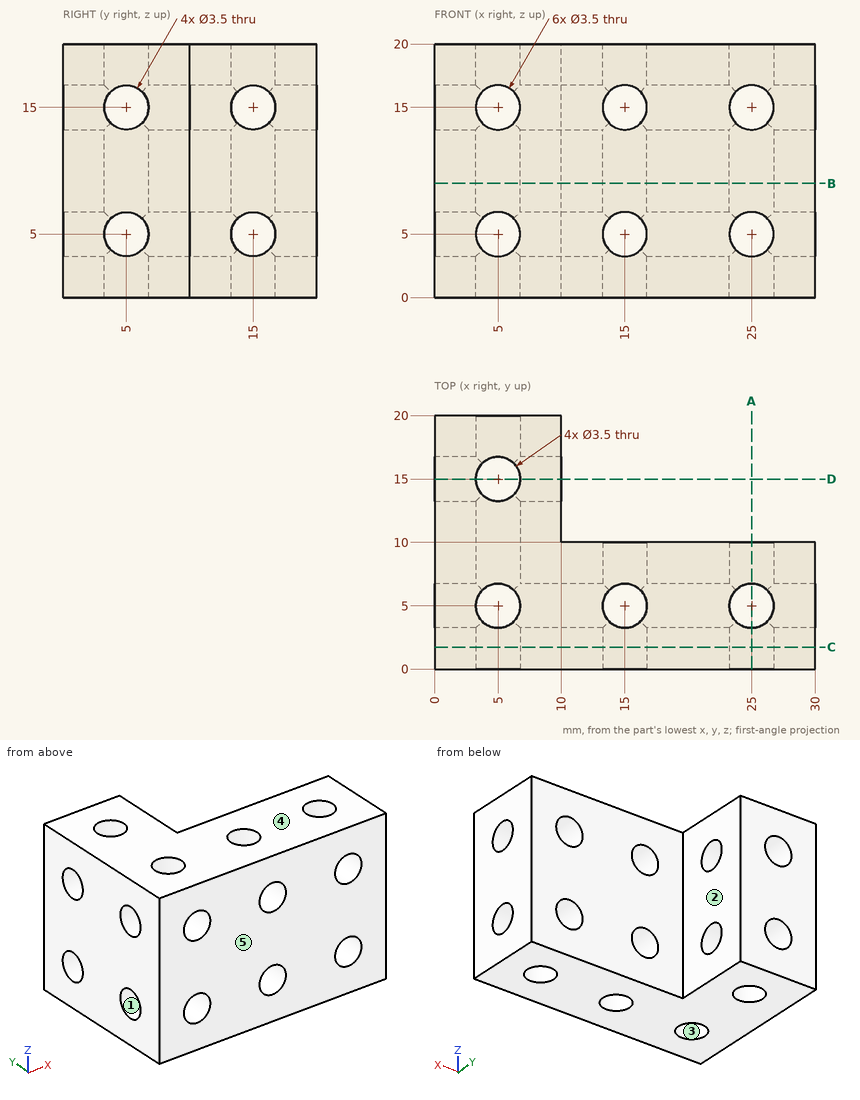
The figure shows three views and two pictorial views of one solid part (mm, origin at its lowest corner). Answer the questions. A direction names the side the tool comes from. Coordinates: 2 decimals unless noted, no trailing zeros. Loops run counter-clockwise (first coordinate to the right, second up) from the corner with the lowest first, then second, coordinate; pieces in that order, holes last. Notation, with made-up numbers: (21.25, 5) -> (51.25, 5) arc R17 ccw to (51.25, 12) -> close; hole circle Ø2 at (24.25, 6). An arc over 180 degrees is marked (long way). Write item = value, one per line. Start each with the question number.
1) Straight lines are drawn through the part: line 1 (Y direction, x = 5, z = 18.35); line 2 (X direction, y = 5, z = 9.75). For each, find the intervals that lie inside material, in ascending order. Write a range as from..to.
2) A cutting plane is placed at C-C (y = 1.75). Give the vertices of the cut face in (x, z), then the cut area to 3 significant figures.
3) Given pin 1 Ø2 at (y, z) = (5, 5) entering from +X; pin 2 Ø4 at (x, z) = (25, 5) entering from +Y, each flat-ended and moving along its own axis, determine where each tip first touches the part or whether it passes through.
4) A tool of negligible diameter and unlimited length cuts with its end or side. For the marked faces 1 and 2, from which of +Z, -Z, +X, -X, +Y, -Y can it reach the whole face along a straight path? Write none if from no direction.
5) A cutting plane is placed at A-A (x = 25). Give the vertices of the cut face in (y, z).
6) A cutting plane is placed at B-B (z = 9). Give the vertices of the cut face in (x, y), then the cut area to 3 significant figures.
7) The mould has two halves that part along Y. Classify the marked faces 3, 4 and 5: released by +Y, released by -Y, zero draft, split by the parting line, or undercut.
Responses:
q1.line_1 = 0..3.25, 6.75..13.25, 16.75..20
q1.line_2 = 0..3.25, 6.75..13.25, 16.75..23.25, 26.75..30
q2.outline = (0, 0) -> (30, 0) -> (30, 20) -> (0, 20) -> close; hole circle Ø3.5 at (5, 5); hole circle Ø3.5 at (5, 15); hole circle Ø3.5 at (15, 5); hole circle Ø3.5 at (15, 15); hole circle Ø3.5 at (25, 5); hole circle Ø3.5 at (25, 15)
q2.area = 542 mm²
q3.pin_1 = through
q3.pin_2 = 10
q4.face_1 = +X, -X
q4.face_2 = +Z, -Z, +X, +Y
q5.outline = (0, 0) -> (3.25, 0) -> (3.25, 3.25) -> (0, 3.25) -> close; (0, 6.75) -> (3.25, 6.75) -> (3.25, 13.25) -> (0, 13.25) -> close; (0, 16.75) -> (3.25, 16.75) -> (3.25, 20) -> (0, 20) -> close; (6.75, 0) -> (10, 0) -> (10, 3.25) -> (6.75, 3.25) -> close; (6.75, 6.75) -> (10, 6.75) -> (10, 13.25) -> (6.75, 13.25) -> close; (6.75, 16.75) -> (10, 16.75) -> (10, 20) -> (6.75, 20) -> close
q6.outline = (0, 0) -> (30, 0) -> (30, 10) -> (10, 10) -> (10, 20) -> (0, 20) -> close; hole circle Ø3.5 at (5, 5); hole circle Ø3.5 at (5, 15); hole circle Ø3.5 at (15, 5); hole circle Ø3.5 at (25, 5)
q6.area = 362 mm²
q7.face_3 = undercut
q7.face_4 = zero draft
q7.face_5 = released by -Y
